from build123d import *

# Parameters (mm, degrees)
F0_R     = 25
F1_DEPTH = 5
F2_W     = 48.538644
F2_H     = 12
F3_DEPTH = 25
F4_W     = 48.538644
F4_H     = 4
F5_DEPTH = 4
F6_R     = 2.5
F7_DEPTH = 31.001


with BuildPart() as f1:
    # F0 (on Top) → F1 (new body)
    with BuildSketch(Plane.XY):
        Circle(F0_R)
    extrude(amount=F1_DEPTH)

    # F2 (on face) → F3 (join)
    with BuildSketch(Plane.XY.offset(5)):
        Rectangle(F2_W, F2_H)
    extrude(amount=F3_DEPTH)

    # F4 (on face) → F5 (cut)
    with BuildSketch(Plane.XY.offset(30)):
        Rectangle(F4_W, F4_H)
    extrude(amount=-F5_DEPTH, mode=Mode.SUBTRACT)

    # F6 (on face) → F7 (cut, through all)
    with BuildSketch(Plane.XZ.offset(6)):
        with Locations((-16.73882, 10.326263)):
            Circle(F6_R)
        with Locations((16.73882, 10.326263)):
            Circle(F6_R)
    extrude(amount=-F7_DEPTH, mode=Mode.SUBTRACT)


solid = f1.part
The model under review builds one solid part; all positions refer to its coordinate system, in mm. A direction names the side the tool comes from. Round coordinates to 2 decimals unless told otherwise and drop trailing zeros. Loops run counter-clockwise (first coordinate to the right, second up) from the corner with the lowest first, then second, coordinate; pieces in that order, holes last. Notation, with made-up numbers: (27, -0.75) -> (71, -0.75) arc R13 cw to (71, 7.25) -> close; hole circle Ø8 at (-18.5, 73.5). An arc over 180 degrees is marked (long way). Write item = value, one per line. Start each with the question number.
Item 1: For faces 5 (the flat face through (24.269, 0, 17)), 6 (the flat face through (0, 6, 17)), 7 (the flat face through (0, -2, 28)), 8 (the flat face through (0, -13, 5)), 9 (the flat face through (0, 0, 0)), list the 3-axis set-ups (+Z, -Z, +X, -X, +Y, -Y) from which the entire face can be reached by the end or side of a thin tool; tool diameter is ignored.
Item 2: Take a section at D-D on z = 2. Give the boundary of the cut face in (x, y), plus the area to 3 significant figures.
Item 3: Take a section at B-B on y = -3. Give the boundary of the cut face in (x, z).
Item 4: Mouldability with a two-part tool opening along X and no side actions: class faces 1 (the cylindrical face through (18.083, -0.084, 12.434)), 2 (the flat face through (0, 0, 26)), 3 (the cylindrical face through (23.846, 7.509, 2.465)), 4 (the flat face through (-24.269, 0, 17)) as released by +X, released by -X, zero draft, split by the parting line, or undercut.
Item 5: Take a section at C-C on y = 7. Give the boundary of the cut face in (x, z).
Item 6: Take a section at A-A on x = 0. Give the boundary of the cut face in (y, z), plus the area to 3 significant figures.
Item 7: To check wall thickness, follow L1, parallel to Y at x = -2, z = 27.75; L2, parallel to Z at x = 21.5, y = -9; L3, parallel to Y at x = 22.5, z = 10. State the ranges of each line that lie inside material, in increasing order.
Item 8: Insertion check: pin 1 (2 mm diameter, centred on x = 9, z = 27, fed in from +Y); pin 2 (6 mm diameter, centred on y = 1, z = 23.5, fed in from +X); pin 3 (4 mm diameter, centred on x = 16.74, z = 10.33, fed in from +Y) (1 decimal); pin 4 (3.5 mm diameter, centred on y = 2.5, z = 23.5, fed in from -X). Each pin has a flat end and moves straight along its axis. Give the tip position at first contact, or say it passes through.
Result:
q1.face_5 = +Z, +X, +Y, -Y
q1.face_6 = +Z, +X, -X, +Y
q1.face_7 = +Z, +X, -X
q1.face_8 = +Z, +X, -X, -Y
q1.face_9 = -Z, +X, -X, +Y, -Y
q2.outline = circle Ø50 at (0, 0)
q2.area = 1,960 mm²
q3.outline = (-24.82, 0) -> (24.82, 0) -> (24.82, 5) -> (24.27, 5) -> (24.27, 30) -> (-24.27, 30) -> (-24.27, 5) -> (-24.82, 5) -> close; hole circle Ø5 at (-16.74, 10.33); hole circle Ø5 at (16.74, 10.33)
q4.face_1 = undercut
q4.face_2 = zero draft
q4.face_3 = split by the parting line
q4.face_4 = released by -X
q5.outline = (-24, 0) -> (24, 0) -> (24, 5) -> (-24, 5) -> close
q6.outline = (-25, 0) -> (25, 0) -> (25, 5) -> (6, 5) -> (6, 30) -> (2, 30) -> (2, 26) -> (-2, 26) -> (-2, 30) -> (-6, 30) -> (-6, 5) -> (-25, 5) -> close
q6.area = 534 mm²
q7.L1 = -6 to -2, 2 to 6
q7.L2 = 0 to 5
q7.L3 = -6 to 6
q8.pin_1 = 6
q8.pin_2 = 24.27
q8.pin_3 = through
q8.pin_4 = -24.27
